Verification items for the finished model (mm, model axes). A direction names the side the tool comes from. Coordinates: 2 decimals unless noted, no trailing zeros. Write each loop counter-clockwise with the first axis right and the second up, starting at its lowest first coordinate (ties: lowest second). Pieces come first, ordered by that corner, then holes. Notation, with made-up numbers: M 82,23 L 123,23 A23 ccw 123,43 Z; hole C 68,39 d11. An arc over 180 degrees is marked long. One line per item, written item: value.
```python
from build123d import *

# Parameters (mm, degrees)
BOSS_EXTRUDE1_DEPTH = 51
CUT_EXTRUDE1_DEPTH  = 6
GREEBLE1_DEPTH      = 52
GREEBLE1_DEPTH_BACK = 52


with BuildPart() as part:
    # Sketch1 → Boss-Extrude1 (new body, symmetric)
    with BuildSketch(Plane(origin=(0, 0, 0), x_dir=(0, 0, -1), z_dir=(1, 0, 0))):
        Polygon((0, 29.75), (0, -29.75), (3, -29.75), (3, -14.75), (5, -14.75), (5, 14.75), (3, 14.75), (3, 29.75), align=None)
    extrude(amount=BOSS_EXTRUDE1_DEPTH, both=True)

    # Sketch3 → Cut-Extrude1 (cut, through all)
    with BuildSketch(Plane.XY):
        with BuildLine():
            Line((23.4, 24), (23.4, 25))
            ThreePointArc((23.4, 25), (25, 26.6), (26.6, 25))
            Line((26.6, 25), (26.6, 24))
            ThreePointArc((26.6, 24), (25, 22.4), (23.4, 24))
        make_face()
        with BuildLine():
            Line((-26.6, 24), (-26.6, 25))
            ThreePointArc((-26.6, 25), (-25, 26.6), (-23.4, 25))
            Line((-23.4, 25), (-23.4, 24))
            ThreePointArc((-23.4, 24), (-25, 22.4), (-26.6, 24))
        make_face()
        with BuildLine():
            Line((26.6, -24), (26.6, -25))
            ThreePointArc((26.6, -25), (25, -26.6), (23.4, -25))
            Line((23.4, -25), (23.4, -24))
            ThreePointArc((23.4, -24), (25, -22.4), (26.6, -24))
        make_face()
        with BuildLine():
            Line((-23.4, -24), (-23.4, -25))
            ThreePointArc((-23.4, -25), (-25, -26.6), (-26.6, -25))
            Line((-26.6, -25), (-26.6, -24))
            ThreePointArc((-26.6, -24), (-25, -22.4), (-23.4, -24))
        make_face()
    extrude(amount=-CUT_EXTRUDE1_DEPTH, mode=Mode.SUBTRACT)

    # Sketch6 → Greeble1 (cut, two sides)
    with BuildSketch(Plane(origin=(0, 0, 0), x_dir=(0, 0, -1), z_dir=(1, 0, 0))) as greeble1_sk:
        with BuildLine():
            ThreePointArc((3, 0), (0.878679656, 0.878679656), (0, 3))
            Line((0, 3), (0, -3))
            ThreePointArc((0, -3), (0.878679656, -0.878679656), (3, 0))
        make_face()
    extrude(amount=GREEBLE1_DEPTH, mode=Mode.SUBTRACT)
    extrude(greeble1_sk.sketch, amount=-GREEBLE1_DEPTH_BACK, mode=Mode.SUBTRACT)


solid = part.part
```
Item 1: Scan lines: line 1 (Y direction, x = -17, z = -3.7); line 2 (Z direction, x = -12, y = -20); line 3 (Y direction, x = -23, z = -0.65). Record each from-to range of solid material in increasing order.
The answers:
line 1: y = -14.75 to 14.75
line 2: z = -3 to 0
line 3: y = -29.75 to -1.14, 1.14 to 29.75
Item 2: Cross-section at B-B, the plane x = -33.5. Enter the section's corners in (y, z).
The answers:
outline: M -29.75,-3 L -14.75,-3 L -14.75,-5 L 14.75,-5 L 14.75,-3 L 29.75,-3 L 29.75,0 L 3,0 A3 ccw 0,-3 A3 ccw -3,0 L -29.75,0 Z
Item 3: Cross-section at C-C, the plane y = 18.5. Enter the section's corners in (x, z), and give its area (3 significant figures).
The answers:
outline: M -51,-3 L 51,-3 L 51,0 L -51,0 Z
area: 306 mm²
Item 4: Access from +Z, -Z, +X, -X, +Y, -Y to the whole of each face (thin tool, end or side, straight path). Record for faces 5 (the face through (25, -26.6, -1.5)), 6 (the face through (1, 22, -3)), 7 (the face through (1, -22, -3)).
The answers:
face 5: +Z, -Z
face 6: -Z, +X, -X, +Y
face 7: -Z, +X, -X, -Y
Item 5: Go/stop test with flat-tipped pins: P1, Ø16.5, axis at x = -16.5, y = -22, coming from the -Z side; P2, Ø3, axis at x = -11, y = -22, coming from the -Z side. Record where each tip stops, or that it passes through.
The answers:
P1: stops at z = -5
P2: stops at z = -3
Item 6: Cross-section at A-A, the plane x = 25. Enter the section's corners in (y, z), and give its area (3 significant figures).
The answers:
outline: M -29.75,-3 L -26.6,-3 L -26.6,0 L -29.75,0 Z; M -22.4,-3 L -14.75,-3 L -14.75,-5 L 14.75,-5 L 14.75,-3 L 22.4,-3 L 22.4,0 L 3,0 A3 ccw 0,-3 A3 ccw -3,0 L -22.4,0 Z; M 26.6,-3 L 29.75,-3 L 29.75,0 L 26.6,0 Z
area: 208 mm²
Item 7: Draft check along X on faces 1 (the face through (51, 0.4, -2.5)), 2 (the face through (1, 14.75, -4)), 3 (the face through (25, -22.4, -1.5)), 4 (the face through (25, 26.6, -1.5)). Enter one of: released by +X, released by -X, zero draft, split by the parting line, or undercut.
The answers:
face 1: released by +X
face 2: zero draft
face 3: undercut
face 4: undercut
Item 8: Cross-section at D-D, the plane z = -3.95. Enter the section's corners in (x, y), and give its area (3 significant figures).
The answers:
outline: M -51,-14.75 L 51,-14.75 L 51,14.75 L -51,14.75 Z
area: 3,010 mm²
